Verification items for the finished model (mm, model axes). Give positions to 0.01 mm unless a question says otherwise; leave off trailing zeros. Loops run counter-clockwise (first coordinate to the right, second up) from the corner with the lowest first, then second, coordinate; pieces in that order, holes last. Notation, with made-up numbers: (11, -24) - (39, -24) arc R27 cw to (39, 15) - close; hole circle Ø7 at (76.5, 21). An arc over 180 degrees is marked (long way). One line per item, written item: value. Start each with the question number.
1. Sectioned sample at A-A (x = 0). Record the cut outline in (y, z) (3 decimals), plus the area to 3 significant figures.
2. Sectioned sample at B-B (y = 1.9). Record the cut outline in (x, z) (3 decimals), plus the area to 3 significant figures.
3. Gauge pin test, flat ends, axial feed: pin 1 (1.5 mm diameter, centred on x = -26.5, y = 2, fed in from -Z); pin 2 (2 mm diameter, centred on x = 13, z = 5.5, fed in from +Y); pin 3 (1.6 mm diameter, centred on x = -34, y = 1, fed in from -Z) (3 decimals); pin 4 (1 mm diameter, centred on x = -22.5, y = 1, fed in from +Z). Record the tip position at first contact, or that the pin passes through.
4. Sectioned sample at D-D (x = 34). Record the cut outline in (y, z) (3 decimals).
5. Sectioned sample at C-C (z = 0). Record the cut outline in (x, y) (3 decimals).
6. Scan lines: L1, parallel to X at y = 2.15, z = 0 (3 decimals); L2, parallel to Z at x = 0, y = 2.2 (3 decimals); L3, parallel to X at y = 2, z = 2. Record each from-to range of solid material in increasing order. Write a range as [from, to].
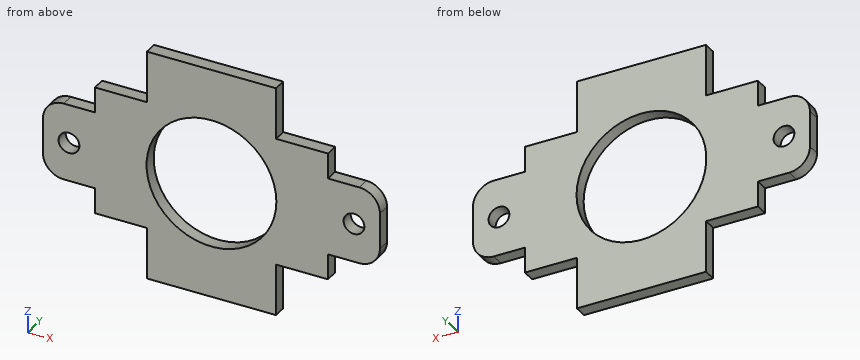
from build123d import *

# Parameters (mm, degrees)
SKETCH1_R           = 15.875
SKETCH1_R_2         = 2.54
BOSS_EXTRUDE1_DEPTH = 3.175


with BuildPart() as part:
    # Sketch1 → Boss-Extrude1 (new body)
    with BuildSketch(Plane(origin=(0, 0, 0), x_dir=(1, 0, 0), z_dir=(0, 1, 0))):
        with BuildLine():
            Line((-28.4999938, 15.7999938), (-28.4999938, 9.525))
            Line((-28.4999938, 9.525), (-36.1199938, 9.525))
            ThreePointArc((-36.1199938, 9.525), (-39.712096248, 8.037102448), (-41.1999938, 4.445))
            Line((-41.1999938, 4.445), (-41.1999938, -4.445))
            ThreePointArc((-41.1999938, -4.445), (-39.712096248, -8.037102448), (-36.1199938, -9.525))
            Line((-36.1199938, -9.525), (-28.4999938, -9.525))
            Line((-28.4999938, -9.525), (-28.4999938, -15.7999938))
            Line((-28.4999938, -15.7999938), (-15.7999938, -15.7999938))
            Line((-15.7999938, -15.7999938), (-15.7999938, -28.4999938))
            Line((-15.7999938, -28.4999938), (15.7999938, -28.4999938))
            Line((15.7999938, -28.4999938), (15.7999938, -15.7999938))
            Line((15.7999938, -15.7999938), (28.4999938, -15.7999938))
            Line((28.4999938, -15.7999938), (28.4999938, -9.525))
            Line((28.4999938, -9.525), (36.1199938, -9.525))
            ThreePointArc((36.1199938, -9.525), (39.712096248, -8.037102448), (41.1999938, -4.445))
            Line((41.1999938, -4.445), (41.1999938, 4.445))
            ThreePointArc((41.1999938, 4.445), (39.712096248, 8.037102448), (36.1199938, 9.525))
            Line((36.1199938, 9.525), (28.4999938, 9.525))
            Line((28.4999938, 9.525), (28.4999938, 15.7999938))
            Line((28.4999938, 15.7999938), (15.7999938, 15.7999938))
            Line((15.7999938, 15.7999938), (15.7999938, 28.4999938))
            Line((15.7999938, 28.4999938), (-15.7999938, 28.4999938))
            Line((-15.7999938, 28.4999938), (-15.7999938, 15.7999938))
            Line((-15.7999938, 15.7999938), (-28.4999938, 15.7999938))
        make_face()
        Circle(SKETCH1_R, mode=Mode.SUBTRACT)
        with Locations((-34.8499938, 0)):
            Circle(SKETCH1_R_2, mode=Mode.SUBTRACT)
        with Locations((34.8499938, 0)):
            Circle(SKETCH1_R_2, mode=Mode.SUBTRACT)
    extrude(amount=BOSS_EXTRUDE1_DEPTH)


solid = part.part
Results are:
1. outline: (0, -28.5) - (3.175, -28.5) - (3.175, -15.875) - (0, -15.875) - close; (0, 15.875) - (3.175, 15.875) - (3.175, 28.5) - (0, 28.5) - close
1. area: 80.2 mm^2
2. outline: (-41.2, -4.445) arc R5.08 ccw to (-36.12, -9.525) - (-28.5, -9.525) - (-28.5, -15.8) - (-15.8, -15.8) - (-15.8, -28.5) - (15.8, -28.5) - (15.8, -15.8) - (28.5, -15.8) - (28.5, -9.525) - (36.12, -9.525) arc R5.08 ccw to (41.2, -4.445) - (41.2, 4.445) arc R5.08 ccw to (36.12, 9.525) - (28.5, 9.525) - (28.5, 15.8) - (15.8, 15.8) - (15.8, 28.5) - (-15.8, 28.5) - (-15.8, 15.8) - (-28.5, 15.8) - (-28.5, 9.525) - (-36.12, 9.525) arc R5.08 ccw to (-41.2, 4.445) - close; hole circle Ø5.08 at (-34.85, 0); hole circle Ø31.75 at (0, 0); hole circle Ø5.08 at (34.85, 0)
2. area: 2,230 mm^2
3. pin 1: stops at z = -15.8
3. pin 2: passes through
3. pin 3: stops at z = -9.525
3. pin 4: stops at z = 15.8
4. outline: (0, -9.525) - (3.175, -9.525) - (3.175, -2.394) - (0, -2.394) - close; (0, 2.394) - (3.175, 2.394) - (3.175, 9.525) - (0, 9.525) - close
5. outline: (-41.2, 0) - (-37.39, 0) - (-37.39, 3.175) - (-41.2, 3.175) - close; (-32.31, 0) - (-15.875, 0) - (-15.875, 3.175) - (-32.31, 3.175) - close; (15.875, 0) - (32.31, 0) - (32.31, 3.175) - (15.875, 3.175) - close; (37.39, 0) - (41.2, 0) - (41.2, 3.175) - (37.39, 3.175) - close
6. L1: x = [-41.2, -37.39], [-32.31, -15.875], [15.875, 32.31], [37.39, 41.2]
6. L2: z = [-28.5, -15.875], [15.875, 28.5]
6. L3: x = [-41.2, -36.42], [-33.28, -15.75], [15.75, 33.28], [36.42, 41.2]
